Build history of the part. All positions in model axes, mm. Give positions to 0.01 mm unless a question says otherwise; leave off trailing zeros. Loops run counter-clockwise (first coordinate to the right, second up) from the corner with the lowest first, then second, coordinate; pieces in that order, holes last. Notation, with made-up numbers: M -1,-6.5 L 22,-6.5 A23 cw 22,30.5 Z; hole C 45.5,-9 d11. An arc over 180 degrees is marked long. Answer as a JSON object with one key per item and string values. Group by question number.
1. Slice it at A-A (x = 5.5). List the corners of the cut face in (y, z) (3 decimals).
2. Slice it at B-B (y = -0.5). List the corners of the cut face in (x, z) (3 decimals).
3. Drill centre lines: line 1 along X through (y, z) = (-1.1, -4); line 2 along Z through (x, y) = (32.5, -1.1) (3 decimals); line 3 along X through (y, z) = (-1.1, -4.25). Where is each one in solid material? Low to high. Write a range as [from, to].
4. Slice it at C-C (z = -4). List the corners of the cut face in (x, y).
from build123d import *

# Parameters (mm, degrees)
SKETCH1_W                   = 37
SKETCH1_H                   = 8
SKETCH1_W_2                 = 34
SKETCH1_H_2                 = 3.25
BASE_FLANGE1_DEPTH          = 1.5
EDGE_FLANGE1_DEPTH          = 8
EDGE_FLANGE1_BEND_DEPTH     = 8
TAP_DRILL_FOR_M3X0_5_TAP1_D = 2.5
FILLET1_START               = -8.5
FILLET1_OUTLINE_W           = 43.3
FILLET1_OUTLINE_H           = 8
FILLET1_OUTLINE_W_2         = 34
FILLET1_OUTLINE_H_2         = 3.25
FILLET1_DEPTH               = 7
FILLET1_START_2             = -1.5
FILLET1_2_OUTLINE_R         = 1.25
FILLET1_2_OUTLINE_W         = 34
FILLET1_2_OUTLINE_H         = 3.25
FILLET1_2_DEPTH             = 1.5


with BuildPart() as part:
    # Base-Flange1: sheet metal written as solids
    # Sketch1 → Base-Flange1 (new body)
    with BuildSketch(Plane(origin=(0, 0, 0), x_dir=(1, 0, 0), z_dir=(0, 1, 0))):
        with Locations((18.5, 4)):
            Rectangle(SKETCH1_W, SKETCH1_H)
        with Locations((18.5, 4)):
            Rectangle(SKETCH1_W_2, SKETCH1_H_2, mode=Mode.SUBTRACT)
    extrude(amount=-BASE_FLANGE1_DEPTH)

    # Edge-Flange1: sheet metal written as solids
    # Edge-Flange1 section (on a plane across the edge) → Edge-Flange1 (add)
    with BuildSketch(Plane(origin=(-1.65, -1.5, 0), x_dir=(1, 0, 0), z_dir=(0, 0, -1))):
        with BuildLine():
            Line((-1.5, 1.65), (-1.5, 7))
            Line((-1.5, 7), (0, 7))
            Line((0, 7), (0, 1.65))
            ThreePointArc((0, 1.65), (0.483273811, 0.483273811), (1.65, 0))
            Line((1.65, 0), (1.65, -1.5))
            ThreePointArc((1.65, -1.5), (-0.577386361, -0.577386361), (-1.5, 1.65))
        make_face()
    extrude(amount=EDGE_FLANGE1_DEPTH)

    # Edge-Flange1 section 2 (on a plane across the edge) → Edge-Flange1 bend (add)
    with BuildSketch(Plane(origin=(38.65, -1.5, -8), x_dir=(-1, 0, 0), z_dir=(0, 0, 1))):
        with BuildLine():
            Line((-1.5, 1.65), (-1.5, 7))
            Line((-1.5, 7), (0, 7))
            Line((0, 7), (0, 1.65))
            ThreePointArc((0, 1.65), (0.483273811, 0.483273811), (1.65, 0))
            Line((1.65, 0), (1.65, -1.5))
            ThreePointArc((1.65, -1.5), (-0.577386361, -0.577386361), (-1.5, 1.65))
        make_face()
    extrude(amount=EDGE_FLANGE1_BEND_DEPTH)

    # Tap Drill for M3x0.5 Tap1 (through all)
    with Locations(Plane(origin=(40.15, 0, 0), x_dir=(0, 0, -1), z_dir=(1, 0, 0))):
        with Locations((4, -5.5)):
            Hole(TAP_DRILL_FOR_M3X0_5_TAP1_D / 2)

    # Fillet1: read off the stored shape, not the designer's step
    # Fillet1 outline → Fillet1 (cut)
    with BuildSketch(Plane(origin=(0, 0, 0), x_dir=(1, 0, 0), z_dir=(0, 1, 0)).offset(FILLET1_START)):
        with Locations((18.5, 4)):
            Rectangle(FILLET1_OUTLINE_W, FILLET1_OUTLINE_H)
        with Locations((18.5, 4)):
            Rectangle(FILLET1_OUTLINE_W_2, FILLET1_OUTLINE_H_2, mode=Mode.SUBTRACT)
    extrude(amount=FILLET1_DEPTH, mode=Mode.SUBTRACT)

    # Fillet1 2 outline → Fillet1 2 (add)
    with BuildSketch(Plane(origin=(0, 0, 0), x_dir=(1, 0, 0), z_dir=(0, 1, 0)).offset(FILLET1_START_2)):
        with BuildLine():
            Line((-9.119911184, 6), (-9.119911184, 2))
            ThreePointArc((-9.119911184, 2), (-8.534124747, 0.585786438), (-7.119911184, 0))
            Line((-7.119911184, 0), (44.119911184, 0))
            ThreePointArc((44.119911184, 0), (45.534124747, 0.585786438), (46.119911184, 2))
            Line((46.119911184, 2), (46.119911184, 6))
            ThreePointArc((46.119911184, 6), (45.534124747, 7.414213562), (44.119911184, 8))
            Line((44.119911184, 8), (-7.119911184, 8))
            ThreePointArc((-7.119911184, 8), (-8.534124747, 7.414213562), (-9.119911184, 6))
        make_face()
        with Locations((-6.119911184, 4)):
            Circle(FILLET1_2_OUTLINE_R, mode=Mode.SUBTRACT)
        with Locations((18.5, 4)):
            Rectangle(FILLET1_2_OUTLINE_W, FILLET1_2_OUTLINE_H, mode=Mode.SUBTRACT)
        with Locations((43.119911184, 4)):
            Circle(FILLET1_2_OUTLINE_R, mode=Mode.SUBTRACT)
    extrude(amount=FILLET1_2_DEPTH)


solid = part.part
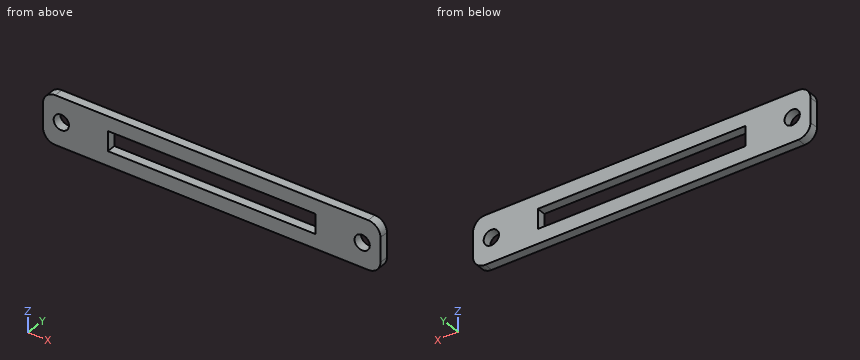
Established:
{
 "1": {"outline": "M -1.5,-8 L 0,-8 L 0,-5.625 L -1.5,-5.625 Z; M -1.5,-2.375 L 0,-2.375 L 0,0 L -1.5,0 Z"},
 "2": {"outline": "M -9.12,-6 A2 ccw -7.12,-8 L 44.12,-8 A2 ccw 46.12,-6 L 46.12,-2 A2 ccw 44.12,0 L -7.12,0 A2 ccw -9.12,-2 Z; hole C -6.12,-4 d2.5; hole M 1.5,-5.625 L 35.5,-5.625 L 35.5,-2.375 L 1.5,-2.375 Z; hole C 43.12,-4 d2.5"},
 "3": {"line 1": "x = [-9.12, -7.37], [-4.87, 1.5], [35.5, 41.87], [44.37, 46.12]", "line 2": "z = [-8, -5.625], [-2.375, 0]", "line 3": "x = [-9.12, -7.34], [-4.9, 1.5], [35.5, 41.9], [44.34, 46.12]"},
 "4": {"outline": "M -9.12,-1.5 L -7.37,-1.5 L -7.37,0 L -9.12,0 Z; M -4.87,-1.5 L 1.5,-1.5 L 1.5,0 L -4.87,0 Z; M 35.5,-1.5 L 41.87,-1.5 L 41.87,0 L 35.5,0 Z; M 44.37,-1.5 L 46.12,-1.5 L 46.12,0 L 44.37,0 Z"}
}
